The listing builds one solid part. Answer for the finished solid, in the listing's coordinates (mm). Face numbers are marked on the shaded views. A direction names the side the tool comes from. Coordinates: 2 decimals unless noted, no trailing zeros. Order: outer loops, then holes, each group sorted by start corner. A loop starts at its lowest first (then second) coordinate and runs counter-clockwise, first axis right, second up. Notation, with made-up numbers: (58.25, 60.5) - (109.25, 60.5) arc R25 cw to (109.25, 82.5) - close; hole circle Ø10 at (77, -13). An arc over 180 degrees is marked (long way). Use one line per item in the form item = value. Start each with the question number.
Item 1: A tool of negligible diameter and unlimited length cuts with its end or side. For the marked faces 1, 2, 3, 4 and 5, from which of +Z, -Z, +X, -X, +Y, -Y can it reach the whole face along a straight path? Write none if from no direction.
Item 2: The mould has two halves that part along X. Classify the marked faces 6, 7 and 8: released by +X, released by -X, zero draft, split by the parting line, or undercut.
Item 3: Section C-C, the plane x = 47 is taken. Write down the section's boundary in (y, z).
Item 4: Section B-B, the plane y = 15 is taken. Write down the section's boundary in (x, z).
Item 5: Each of these flat-tipped pins is pushed along its axis until it touches: pin 1 Ø15 at (x, y) = (40, 36.5) entering from -Z; pin 2 Ø6.5 at (x, z) = (63.5, 47.5) entering from -Y; pin 3 Ø8.5 at (x, y) = (25.82, 27.61) entering from +Z; pin 4 Ø4 at (y, z) = (24, 3.5) entering from +X. Where does it stop, or does it pass through?
Item 6: Consider line 1 along Z through (x, y) = (5, 22); line 2 along Z through (x, y) = (32, 38.5); line 3 along X through (y, z) = (2, 37). Determine where each line is inside the solid, lowest interval first. Write a range as [from, to].
Item 7: Section A-A, the plane x = 62.5 is taken. Write down the section's boundary in (y, z).
Item 8: Section D-D, the plane y = 46 is taken. Write down the section's boundary in (x, z).
from build123d import *

# Parameters (mm, degrees)
F2_DEPTH = 50.8
F1_R     = 7.203181
F1_R_2   = 9.266269
F3_DEPTH = 88.9
F4_W     = 12.7
F4_H     = 12.7
F5_DEPTH = 38.1
F7_DEPTH = 76.2


with BuildPart() as f2:
    # F0 (on Front) → F2 (new body)
    with BuildSketch(Plane.XZ):
        Polygon((0, 0), (12.7, 0), (12.7, 8.135938), (76.2, 8.135938), (76.2, 50.983995), (38.1, 50.8), (38.1, 17.396355), (0, 17.396355), align=None)
    extrude(amount=-F2_DEPTH)

    # F1 (on Top) → F3 (cut)
    with BuildSketch(Plane.XY):
        with Locations((25.821837, 27.612405)):
            Circle(F1_R)
        with Locations((60.502268, 20.073181)):
            Circle(F1_R_2)
    extrude(amount=F3_DEPTH, mode=Mode.SUBTRACT)

    # F4 (on face) → F5 (join)
    with BuildSketch(Plane.YZ.offset(76.2)):
        with Locations((44.45, 44.633995)):
            Rectangle(F4_W, F4_H)
    extrude(amount=-F5_DEPTH)

    # F6 (on Right) → F7 (cut)
    with BuildSketch(Plane.YZ):
        Polygon((38.1, 51.342876), (0, 50.983995), (0, 38.283995), (38.1, 38.283995), align=None)
    extrude(amount=F7_DEPTH, mode=Mode.SUBTRACT)


solid = f2.part
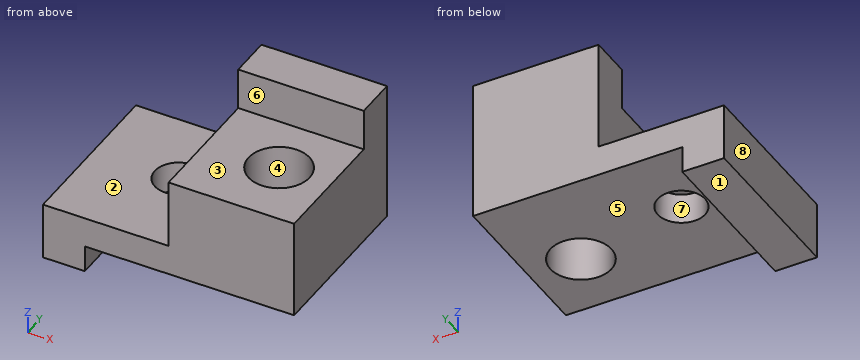
Response:
q1.face_1 = -Z, +X, -X, +Y, -Y
q1.face_2 = +Z, -X, +Y, -Y
q1.face_3 = +Z, +X, -X, -Y
q1.face_4 = +Z, -Z
q1.face_5 = -Z, +X, +Y, -Y
q2.face_6 = zero draft
q2.face_7 = undercut
q2.face_8 = released by -X
q3.outline = (0, 8.14) - (50.8, 8.14) - (50.8, 50.98) - (38.1, 50.98) - (38.1, 38.28) - (0, 38.28) - close
q4.outline = (0, 0) - (12.7, 0) - (12.7, 8.14) - (52.75, 8.14) - (52.75, 38.28) - (38.1, 38.28) - (38.1, 17.4) - (0, 17.4) - close; (68.26, 8.14) - (76.2, 8.14) - (76.2, 38.28) - (68.26, 38.28) - close
q5.pin_1 = 8.14
q5.pin_2 = 38.1
q5.pin_3 = through
q5.pin_4 = 12.7
q6.line_1 = [0, 17.4]
q6.line_2 = [8.14, 17.4]
q6.line_3 = [38.1, 76.2]
q7.outline = (0, 8.14) - (11.02, 8.14) - (11.02, 38.28) - (0, 38.28) - close; (29.12, 8.14) - (50.8, 8.14) - (50.8, 50.98) - (38.1, 50.98) - (38.1, 38.28) - (29.12, 38.28) - close
q8.outline = (0, 0) - (12.7, 0) - (12.7, 8.14) - (76.2, 8.14) - (76.2, 50.98) - (38.1, 50.98) - (38.1, 17.4) - (0, 17.4) - close
